CAD build for the part. Positions are in the model's coordinates, mm. Give positions to 0.01 mm unless a question says otherwise; leave off trailing zeros. Order: outer loops, then holes, each group sorted by start corner. A loop starts at its lowest first (then second) coordinate and runs counter-clockwise, first axis right, second up.
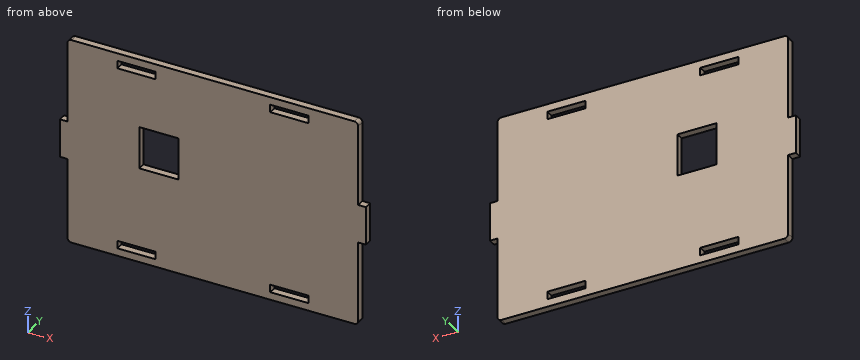
Solid Edge part; units mm, degrees
sketch "Sketch1" plane through (0, 0, 0) normal (0, -1, 0) x (1, 0, 0)
  line L0 (40, -27) -> (40, 27)
  line L1 (40, 27) -> (-40, 27)
  line L2 (-40, 27) -> (-40, -27)
  line L3 (-40, -27) -> (40, -27)
extrude "Protrusion1" add sketch "Sketch1" along normal blind 2
sketch "Sketch2" plane through (0, 0, 0) normal (0, -1, 0) x (1, 0, 0)
  line L0 (-25, 23) -> (-15, 23)
  line L1 (-15, 23) -> (-15, 25)
  line L2 (-15, 25) -> (-25, 25)
  line L3 (-25, 25) -> (-25, 23)
extrude "ExtrudedCutout_1" cut sketch "Sketch2" along normal blind 2
sketch "Sketch3" plane through (0, 0, 0) normal (0, -1, 0) x (1, 0, 0)
  line L0 (25, 25) -> (15, 25)
  line L1 (15, 25) -> (15, 23)
  line L2 (15, 23) -> (25, 23)
  line L3 (25, 23) -> (25, 25)
extrude "ExtrudedCutout_2" cut sketch "Sketch3" along normal blind 2
sketch "Sketch4" plane through (0, 0, 0) normal (0, -1, 0) x (1, 0, 0)
  line L0 (15, -25) -> (25, -25)
  line L1 (25, -25) -> (25, -23)
  line L2 (25, -23) -> (15, -23)
  line L3 (15, -23) -> (15, -25)
extrude "ExtrudedCutout_3" cut sketch "Sketch4" along normal blind 2
sketch "Sketch5" plane through (0, 0, 0) normal (0, -1, 0) x (1, 0, 0)
  line L0 (-15, -23) -> (-25, -23)
  line L1 (-25, -23) -> (-25, -25)
  line L2 (-25, -25) -> (-15, -25)
  line L3 (-15, -25) -> (-15, -23)
extrude "ExtrudedCutout_4" cut sketch "Sketch5" along normal blind 2
sketch "Sketch6" plane through (0, 0, 0) normal (0, -1, 0) x (1, 0, 0)
  line L0 (-38, -27) -> (-38, -5)
  line L1 (-38, -5) -> (-40, -5)
  line L2 (-40, -5) -> (-40, -27)
  line L3 (-40, -27) -> (-38, -27)
extrude "ExtrudedCutout_5" cut sketch "Sketch6" along normal blind 2
sketch "Sketch7" plane through (0, 0, 0) normal (0, -1, 0) x (1, 0, 0)
  line L0 (-38, 5) -> (-38, 27)
  line L1 (-38, 27) -> (-40, 27)
  line L2 (-40, 27) -> (-40, 5)
  line L3 (-40, 5) -> (-38, 5)
extrude "ExtrudedCutout_6" cut sketch "Sketch7" along normal blind 2
sketch "Sketch8" plane through (0, 0, 0) normal (0, -1, 0) x (1, 0, 0)
  line L0 (38, -5) -> (38, -27)
  line L1 (38, -27) -> (40, -27)
  line L2 (40, -27) -> (40, -5)
  line L3 (40, -5) -> (38, -5)
extrude "ExtrudedCutout_7" cut sketch "Sketch8" along normal blind 2
sketch "Sketch9" plane through (0, 0, 0) normal (0, -1, 0) x (1, 0, 0)
  line L0 (38, 27) -> (38, 5)
  line L1 (38, 5) -> (40, 5)
  line L2 (40, 5) -> (40, 27)
  line L3 (40, 27) -> (38, 27)
extrude "ExtrudedCutout_8" cut sketch "Sketch9" along normal blind 2
sketch "Sketch10" plane through (0, 0, 0) normal (0, -1, 0) x (1, 0, 0)
  line L0 (-19.25, -2) -> (-9, -2)
  line L1 (-9, -2) -> (-9, 9)
  line L2 (-9, 9) -> (-19.25, 9)
  line L3 (-19.25, 9) -> (-19.25, -2)
extrude "ExtrudedCutout_9" cut sketch "Sketch10" along normal blind 2
fillet "Round_1" radius 1 4 edges at (38, -1, -27) (38, -1, 27) (-38, -1, 27) (-38, -1, -27)
properties material "Acrylic, high impact grade"
Item 1: Slice it at B-B (z = 3.5). Give the cut face in (x, y), and give its area (4 significant figures).
Item 2: Slice it at C-C (x = 22.5). Give the cut face in (y, z).
Item 3: Slice it at D-D (y = -1.3). State how many separate pieces and enclosed holes the cut face has, and give its area (3 significant figures).
Item 4: Wall check: L1, parallel to Z at x = -21.5, y = -0.45; L2, parallel to X at y = -0.1, z = -24; L3, parallel to X at y = -1.75, z = 3.5. Give the ranges that are in metal, low to high.
Item 5: Drop flat-ended pins along their axis: pin 1 Ø1 at (y, z) = (-0.5, -20.5) entering from -X; pin 2 Ø0.6 at (y, z) = (-1.5, 23.5) entering from +X. Give the stop position or say it passes through.
Item 6: Slice it at A-A (x = -11). Give the cut face in (y, z).
A:
1. outline: (-40, -2) - (-19.25, -2) - (-19.25, 0) - (-40, 0) - close; (-9, -2) - (40, -2) - (40, 0) - (-9, 0) - close
1. area: 139.5 mm2
2. outline: (-2, -27) - (0, -27) - (0, -25) - (-2, -25) - close; (-2, -23) - (0, -23) - (0, 23) - (-2, 23) - close; (-2, 25) - (0, 25) - (0, 27) - (-2, 27) - close
3. separate pieces: 1
3. enclosed holes: 5
3. area: 3,950 mm2
4. L1: z = -27 to -25, -23 to 23, 25 to 27
4. L2: x = -38 to -25, -15 to 15, 25 to 38
4. L3: x = -40 to -19.25, -9 to 40
5. pin 1: stops at x = -38
5. pin 2: stops at x = 38
6. outline: (-2, -27) - (0, -27) - (0, -2) - (-2, -2) - close; (-2, 9) - (0, 9) - (0, 27) - (-2, 27) - close
